from build123d import *

# Parameters (mm, degrees)
BOSS_EXTRUDE2_DEPTH  = 9.525
BOSS_EXTRUDE4_DEPTH  = 38.1
SKETCH5_R            = 6.35
BOSS_EXTRUDE6_DEPTH  = 3.175
SKETCH5_6_W          = 28.575
SKETCH5_6_H          = 4.7625
BOSS_EXTRUDE10_DEPTH = 4.7625
SKETCH5_7_R          = 6.35
CUT_EXTRUDE1_DEPTH   = 73.470722537
FILLET1_R            = 9.525
FILLET4_R            = 1.905
FILLET5_R            = 1.905


with BuildPart() as part:
    # Sketch1 → Boss-Extrude2 (new body)
    with BuildSketch(Plane(origin=(0, 0, 0), x_dir=(1, 0, 0), z_dir=(0, 1, 0))):
        with BuildLine():
            Line((-38.1, -25.4), (38.1, -25.4))
            ThreePointArc((38.1, -25.4), (42.590128061, -23.540128061), (44.45, -19.05))
            Line((44.45, -19.05), (44.45, 25.4))
            Line((44.45, 25.4), (-44.45, 25.4))
            Line((-44.45, 25.4), (-44.45, -19.05))
            ThreePointArc((-44.45, -19.05), (-42.590128061, -23.540128061), (-38.1, -25.4))
        make_face()
    extrude(amount=BOSS_EXTRUDE2_DEPTH)

    # Sketch4 → Boss-Extrude4 (add)
    with BuildSketch(Plane(origin=(0, 9.525, 0), x_dir=(1, 0, 0), z_dir=(0, 1, 0))):
        Polygon((30.1625, 25.4), (30.1625, -6.35), (-30.1625, -6.35), (-30.1625, 25.4), (-20.6375, 25.4), (-20.6375, 6.35), (20.6375, 6.35), (20.6375, 25.4), align=None)
    extrude(amount=BOSS_EXTRUDE4_DEPTH)

    # Sketch5 → Boss-Extrude6 (add)
    with BuildSketch(Plane.XY.offset(6.35)):
        with BuildLine():
            Line((-14.2875, 14.2875), (-14.2875, 28.575))
            ThreePointArc((-14.2875, 28.575), (0, 42.8625), (14.2875, 28.575))
            Line((14.2875, 28.575), (14.2875, 14.2875))
            Line((14.2875, 14.2875), (-14.2875, 14.2875))
        make_face()
        with Locations((0, 28.575)):
            Circle(SKETCH5_R, mode=Mode.SUBTRACT)
    extrude(amount=BOSS_EXTRUDE6_DEPTH)

    # Sketch5_6 → Boss-Extrude10 (add)
    with BuildSketch(Plane.XY.offset(6.35)):
        with Locations((0, 11.90625)):
            Rectangle(SKETCH5_6_W, SKETCH5_6_H)
    extrude(amount=BOSS_EXTRUDE10_DEPTH)

    # Sketch5_7 → Cut-Extrude1 (cut, through all)
    with BuildSketch(Plane.XY.offset(6.35)):
        with Locations((0, 28.575)):
            Circle(SKETCH5_7_R)
    extrude(amount=-CUT_EXTRUDE1_DEPTH, mode=Mode.SUBTRACT)

    # Fillet1
    fillet1_edges = [part.edges().sort_by_distance(p)[0] for p in [
        (-30.1625, 9.525, -9.525),
        (30.1625, 9.525, -9.525),
    ]]
    fillet(fillet1_edges, radius=FILLET1_R)

    # Fillet4
    fillet4_edges = [part.edges().sort_by_distance(p)[0] for p in [
        (0, 42.8625, 6.35),
        (14.2875, 19.05, 6.35),
        (-14.2875, 19.05, 6.35),
    ]]
    fillet(fillet4_edges, radius=FILLET4_R)

    # Fillet5
    fillet5_edges = [part.edges().sort_by_distance(p)[0] for p in [
        (27.94, 9.525, 6.35),
        (-14.845461582, 9.525, 6.907961582),
        (14.845461582, 9.525, 6.907961582),
        (-27.94, 9.525, 6.35),
        (-14.2875, 9.525, 9.68375),
        (14.2875, 9.525, 9.68375),
    ]]
    fillet(fillet5_edges, radius=FILLET5_R)


solid = part.part
Model file for the job. Use its own axes, mm. A direction names the side the tool comes from. Give positions to 0.01 mm unless a question says otherwise; leave off trailing zeros. Write each loop counter-clockwise with the first axis right and the second up, starting at its lowest first coordinate (ties: lowest second). Pieces come first, ordered by that corner, then holes. Notation, with made-up numbers: M -24.5,4.5 L -16.5,4.5 A11 cw -16.5,22.5 Z; hole C -16,45 d8. An arc over 180 degrees is marked long. One line per item, written item: value. Start each with the question number.
Q1. Probe probe 1 along Y at (x, z) = (0, 8.1) (3 decimals); probe 2 along Y at (x, z) = (0, -1) (3 decimals); probe 3 along X at (y, z) = (28.5, -20). List the from-to ranges inside material, lowest first. Write a range as [from, to].
Q2. Two-plate mould, pull along X, no slides. Class faces 1 (the cylindrical face through (14.831, 19.882, 6.923)), 2 (the cylindrical face through (25.16, 10.07, 6.92)), 3 (the flat face through (-20.638, 28, -16)), 4 (the cylindrical face through (-14.831, 20.123, 6.923)): +X half, -X half, draft (parallel to the pull), parting line (faces both ways), or undercut.
Q3. Drop flat-ended pins along their axis: pin 1 Ø5.5 at (x, z) = (-1, -14) entering from +Y (3 decimals); pin 2 Ø8.5 at (x, y) = (6, 31) entering from +Z (3 decimals); pin 3 Ø8.5 at (y, z) = (32.5, -2) entering from -X. Give the stop position or say it passes through.
Q4. 3-axis set-ups, long thin cutter, end or side, ignore diameter. For faces 5 (the flat face through (-15, 37, 6.35)), 6 (the flat face through (0, 12, 11.112)), 7 (the flat face through (-30.162, 33, -9)), 8 (the cylindrical face through (-25.49, 10.07, 6.92)): which of +Z, -Z, +X, -X, +Y, -Y reach the whole face in a straight line?
Q5. Saw through at B-B, the plane x = -19.5. Write the cut outline in (y, z) (3 decimals), plus the area to 3 significant figures.
Output values:
1. probe 1: y = [0, 22.225], [34.925, 42.869]
1. probe 2: y = [0, 22.225], [34.925, 47.625]
1. probe 3: x = [-30.16, -20.64], [20.64, 30.16]
2. face 1: +X half
2. face 2: draft
2. face 3: undercut
2. face 4: -X half
3. pin 1: stops at y = 9.525
3. pin 2: stops at z = 9.525
3. pin 3: stops at x = -30.16
4. face 5: +Z, +Y
4. face 6: +Z, +X, -X, +Y
4. face 7: +Z, -Z, -X, +Y
4. face 8: +Z, -X, +Y
5. outline: M 0,-25.4 L 9.525,-25.4 L 9.525,-6.35 L 47.625,-6.35 L 47.625,6.35 L 11.43,6.35 A1.905 cw 9.525,8.255 L 9.525,25.4 L 0,25.4 Z
5. area: 969 mm²
